```python
from build123d import *

# Parameters (mm, degrees)
IZIM1_R                     = 1.5
Y_KSEKLIK_EKSTR_ZYON1_DEPTH = 6.6
IZIM3_W                     = 2
IZIM3_H                     = 2
Y_KSEKLIK_EKSTR_ZYON3_DEPTH = 6.6
IZIM4_W                     = 2
IZIM4_H                     = 2
Y_KSEKLIK_EKSTR_ZYON4_DEPTH = 2


with BuildPart() as part:
    # Çizim1 → Yükseklik-Ekstrüzyon1 (new body)
    # profile 1 of 2: a face of its own
    with BuildSketch(Plane(origin=(0, 0, 0), x_dir=(0, 1, 0), z_dir=(0, 0, 1))):
        Polygon((0, 50), (0, 0), (25.5, 0), (25.5, 7.6), (25.5, 31.5), (25.5, 50), align=None)
        with Locations(Location((2.5, 2.5, 0), (0, 0, 270))):
            Circle(IZIM1_R, mode=Mode.SUBTRACT)
        with Locations(Location((2.5, 47.5, 0), (0, 0, 270))):
            Circle(IZIM1_R, mode=Mode.SUBTRACT)
    # profile 2 of 2: a face of its own
    with BuildSketch(Plane(origin=(0, 0, 0), x_dir=(0, 1, 0), z_dir=(0, 0, 1))):
        Polygon((25.5, 31.5), (25.5, 7.6), (90.3, 7.6), (90.3, 68.7), (66.3, 68.7), (66.3, 31.5), align=None)
    extrude(amount=Y_KSEKLIK_EKSTR_ZYON1_DEPTH)

    # Çizim3 → Yükseklik-Ekstrüzyon3 (add)
    with BuildSketch(Plane(origin=(0, 0, 0), x_dir=(0, 1, 0), z_dir=(0, 0, 1))):
        with Locations((65.3, 32.5)):
            Rectangle(IZIM3_W, IZIM3_H)
        with Locations((91.3, 32.5)):
            Rectangle(IZIM3_W, IZIM3_H)
        with Locations((65.3, 6.6)):
            Rectangle(IZIM3_W, IZIM3_H)
    extrude(amount=Y_KSEKLIK_EKSTR_ZYON3_DEPTH)

    # Çizim4 → Yükseklik-Ekstrüzyon4 (add)
    with BuildSketch(Plane.XY.offset(6.6)):
        with Locations((-32.5, 91.3)):
            Rectangle(IZIM4_W, IZIM4_H)
        with Locations((-32.5, 65.3)):
            Rectangle(IZIM4_W, IZIM4_H)
        with Locations((-6.6, 65.3)):
            Rectangle(IZIM4_W, IZIM4_H)
    extrude(amount=Y_KSEKLIK_EKSTR_ZYON4_DEPTH)


solid = part.part
```
Design review of the part built by this model. Coordinates are the model's own, in mm. A direction names the side the tool comes from. Round coordinates to 2 decimals unless told otherwise and drop trailing zeros. Write each loop counter-clockwise with the first axis right and the second up, starting at its lowest first coordinate (ties: lowest second). Pieces come first, ordered by that corner, then holes.
Item 1: For probe 1 along Y at (x, z) = (-47.5, 2); probe 2 along Y at (x, z) = (-42.5, 0.5); probe 3 along Y at (x, z) = (-2.5, 4), list the stretches that pass through material, from the lowest coordinate up.
Item 2: We need section A-A on x = -47.5. Write out the cut boundary in (y, z), and give its area (3 significant figures).
Item 3: The part is to be moulded in two halves that separate along Y. For faces 1 (the flat face through (-33, 92.3, 4)), 2 (the flat face through (-33, 66.3, 8)), 3 (the flat face through (-51, 66.3, 3)), 4 (the flat face through (-33, 65, 8.6)), say which applies: +Y half, -Y half, draft (parallel to the pull), parting line (faces both ways), or undercut.
Item 4: We need section D-D on x = -2.5. Write out the cut boundary in (y, z), and give its area (4 significant figures).
Item 5: We need section C-C on y = 2.5. Write out the cut boundary in (x, z).
Item 6: For faces 5 (the flat face through (-7.6, 45, 3)), 6 (the flat face through (-7.6, 65, 8)), 7 (the flat face through (-32, 64.3, 4)), 8 (the flat face through (-31.5, 91, 4)), list the 3-axis set-ups (+Z, -Z, +X, -X, +Y, -Y) from which the entire face can be reached by the end or side of a thin tool; tool diameter is ignored.
Item 7: Clearance check with flat-ended pins moving along their axes: pin 1 Ø1 at (x, z) = (-7, 5) entering from +Y; pin 2 Ø2 at (y, z) = (76, 6) entering from +X; pin 3 Ø0.6 at (y, z) = (91.5, 4.5) entering from -X; pin 4 Ø6 at (x, y) = (-55, 11.5) entering from +Z. State where each tip first meets the part, or that it passes through.
Item 8: We need section B-B on z = 2.5. Write out the cut boundary in (x, y).
Returned:
1. probe 1: y = 0 to 1, 4 to 25.5, 66.3 to 90.3
1. probe 2: y = 0 to 25.5, 66.3 to 90.3
1. probe 3: y = 0 to 1, 4 to 25.5
2. outline: (0, 0) - (1, 0) - (1, 6.6) - (0, 6.6) - close; (4, 0) - (25.5, 0) - (25.5, 6.6) - (4, 6.6) - close; (66.3, 0) - (90.3, 0) - (90.3, 6.6) - (66.3, 6.6) - close
2. area: 307 mm2
3. face 1: +Y half
3. face 2: undercut
3. face 3: undercut
3. face 4: draft
4. outline: (0, 0) - (1, 0) - (1, 6.6) - (0, 6.6) - close; (4, 0) - (25.5, 0) - (25.5, 6.6) - (4, 6.6) - close
4. area: 148.5 mm2
5. outline: (-50, 0) - (-49, 0) - (-49, 6.6) - (-50, 6.6) - close; (-46, 0) - (-4, 0) - (-4, 6.6) - (-46, 6.6) - close; (-1, 0) - (0, 0) - (0, 6.6) - (-1, 6.6) - close
6. face 5: +Z, -Z, +X
6. face 6: +Z, +Y, -Y
6. face 7: +Z, -Z, -X
6. face 8: +Z, -Z, +X, +Y
7. pin 1: stops at y = 66.3
7. pin 2: stops at x = -7.6
7. pin 3: stops at x = -33.5
7. pin 4: passes through
8. outline: (-68.7, 66.3) - (-33.5, 66.3) - (-33.5, 64.3) - (-31.5, 64.3) - (-31.5, 25.5) - (-50, 25.5) - (-50, 0) - (0, 0) - (0, 25.5) - (-7.6, 25.5) - (-7.6, 64.3) - (-5.6, 64.3) - (-5.6, 66.3) - (-7.6, 66.3) - (-7.6, 90.3) - (-31.5, 90.3) - (-31.5, 92.3) - (-33.5, 92.3) - (-33.5, 90.3) - (-68.7, 90.3) - close; hole circle Ø3 at (-47.5, 2.5); hole circle Ø3 at (-2.5, 2.5)
